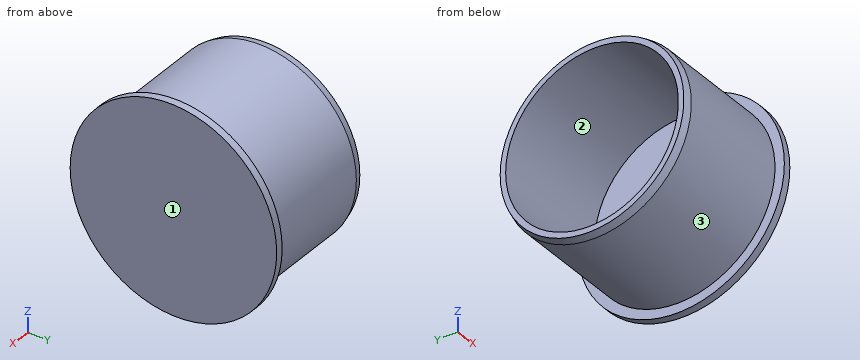
Autodesk Fusion 360 part; units mm, degrees
sketch "Skizze1" plane through (0, 0, 0) normal (0, 0, 1) x (1, 0, 0)
  line L0 (0, 0) -> (0, 27.5)
  line L1 (0, 27.5) -> (-2, 27.5)
  line L2 (-2, 27.5) -> (-2, 25)
  line L3 (-2, 25) -> (-32.5, 25)
  line L4 (-32.5, 25) -> (-34.5, 24.4641)
  line L5 (-34.5, 24.4641) -> (-34.5, 23)
  line L6 (-34.5, 23) -> (-2, 23)
  line L7 (-2, 23) -> (-2, 0)
  line L8 (-2, 0) -> (0, 0)
  dimension "d2" = 27.5
  dimension "d3" = 32.5
  dimension "d4" = 2
  dimension "d5" = 23
  dimension "d6" = 25
  dimension "d7" = 15
  dimension "d8" = 2
revolve "Drehen1" add sketch "Skizze1" angle 360 about axis through (1.75, 0, 0) along (1, 0, 0)
equation "d2 = ( 55 / 2 ) * 1 mm"
equation "d5 = ( 46 / 2 ) * 1 mm"
equation "d6 = ( 50 / 2 ) * 1 mm"
Build history of the part. All positions in model axes, mm. Face numbers are marked on the shaded views. Give positions to 0.01 mm unless a question says otherwise; leave off trailing zeros. Loops run counter-clockwise (first coordinate to the right, second up) from the corner with the lowest first, then second, coordinate; pieces in that order, holes last.
Item 1: Flat gauge pins, fed straight in: pin 1 (2 mm diameter, centred on x = -17.5, y = 10, fed in from -Z); pin 2 (5 mm diameter, centred on x = -22, z = 17.5, fed in from +Y); pin 3 (12 mm diameter, centred on x = -28, y = 15.5, fed in from +Z). Where does each tip first touch, or does it go through?
Answers follow:
pin 1: stops at z = -23.32
pin 2: stops at y = 20
pin 3: stops at z = 23.12
Item 2: Slice it at A-A, the plane y = 0. List the corners of the cut face in (x, z), and give its area (3 significant figures).
Answers follow:
outline: (-34.5, -24.46) - (-32.5, -25) - (-2, -25) - (-2, -27.5) - (0, -27.5) - (0, 27.5) - (-2, 27.5) - (-2, 25) - (-32.5, 25) - (-34.5, 24.46) - (-34.5, 23) - (-2, 23) - (-2, -23) - (-34.5, -23) - close
area: 239 mm2
Item 3: Drill centre lines: line 1 (Z direction, x = -25, y = 0); line 2 (X direction, y = 6.5, z = -18); line 3 (Y direction, x = -6, z = 0.5) (3 decimals). Where is each one in solid material? Low to high.
Answers follow:
line 1: z = -25 to -23, 23 to 25
line 2: x = -2 to 0
line 3: y = -24.995 to -22.995, 22.995 to 24.995
Item 4: Pull direction Y, two halves, no side cores. Call the marked faces 1, 2 and 3: released by +Y, released by -Y, zero draft, split by the parting line, or undercut.
Answers follow:
face 1: zero draft
face 2: undercut
face 3: split by the parting line
Item 5: Slice it at C-C, the plane x = -27. List the corners of the cut face in (y, z), and give its area (3 significant figures).
Answers follow:
outline: circle Ø50 at (0, 0); hole circle Ø46 at (0, 0)
area: 302 mm2
